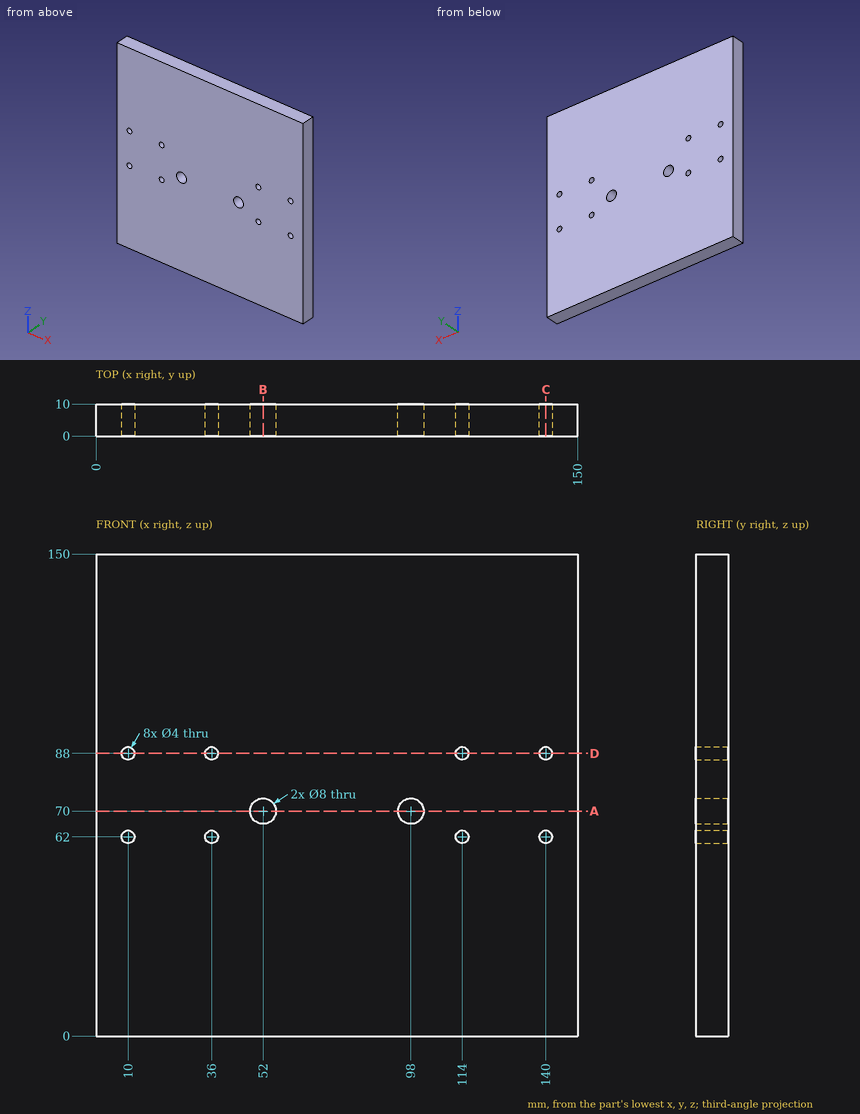
Check sheet for the drawn part. Datum: minimum x, y, z corner. Units: mm. Give positions to 0.01 mm unless a question says otherwise; leave off trailing zeros. Loops run counter-clockwise (first coordinate to the right, second up) from the corner with the lowest first, then second, coordinate; pieces in that order, holes last. Notation, with made-up numbers: M 40,-6.75 L 46,-6.75 A27 ccw 46,22.25 Z; hole C 72,-37 d10. An arc over 180 degrees is marked long. Answer as CSV lines item,"result".
Item 1: Depth check by flat-ended pin: pin 1 Ø3 at (x, z) = (10, 88) entering from +Y. Enter the tip coordinate at first touch or a pass-through.
Reply:
pin 1,"through"
Item 2: Scan lines: L1, parallel to X at y = 2.75, z = 70; L2, parallel to X at y = 4.25, z = 62; L3, parallel to Z at x = 36, y = 5.25. Record each from-to range of solid material in increasing order.
Reply:
L1,"0 to 48, 56 to 94, 102 to 150"
L2,"0 to 8, 12 to 34, 38 to 112, 116 to 138, 142 to 150"
L3,"0 to 60, 64 to 86, 90 to 150"
Item 3: Sectioned sample at B-B, the plane x = 52. Enter the section's corners in (y, z).
Reply:
outline,"M 0,0 L 10,0 L 10,66 L 0,66 Z; M 0,74 L 10,74 L 10,150 L 0,150 Z"
Item 4: Sectioned sample at A-A, the plane z = 70. Enter the section's corners in (x, y), then the cut area to 3 significant figures.
Reply:
outline,"M 0,0 L 48,0 L 48,10 L 0,10 Z; M 56,0 L 94,0 L 94,10 L 56,10 Z; M 102,0 L 150,0 L 150,10 L 102,10 Z"
area,"1,340 mm^2"
Item 5: Sectioned sample at C-C, the plane x = 140. Enter the section's corners in (y, z), then the cut area to 3 significant figures.
Reply:
outline,"M 0,0 L 10,0 L 10,60 L 0,60 Z; M 0,64 L 10,64 L 10,86 L 0,86 Z; M 0,90 L 10,90 L 10,150 L 0,150 Z"
area,"1,420 mm^2"
Item 6: Sectioned sample at D-D, the plane z = 88. Enter the section's corners in (x, y).
Reply:
outline,"M 0,0 L 8,0 L 8,10 L 0,10 Z; M 12,0 L 34,0 L 34,10 L 12,10 Z; M 38,0 L 112,0 L 112,10 L 38,10 Z; M 116,0 L 138,0 L 138,10 L 116,10 Z; M 142,0 L 150,0 L 150,10 L 142,10 Z"
